```python
from build123d import *

# Parameters (mm, degrees)
F2_R     = 4.7625
F3_DEPTH = 5.08
F4_SIZE  = 0.381
F5_R     = 0.534423
F6_DEPTH = 25.4


with BuildPart() as f1:
    # F0 (on Front) → F1 (revolve)
    with BuildSketch(Plane.XZ):
        Polygon((0, 1.6002), (0, 0), (0, -3.2004), (12.659507, -3.2004), (12.659507, -1.6002), (10.346893, -1.6002), (10.346893, 0), (12.7, 0), (12.7, 1.6002), align=None)
    revolve(axis=Axis((0, 0, 0.8001), (0, 0, 1)))

    # F2 (on face) → F3 (cut)
    with BuildSketch(Plane.XY.offset(1.6002)):
        with Locations((0, -3.9624)):
            Circle(F2_R)
    extrude(amount=-F3_DEPTH, mode=Mode.SUBTRACT)

    # F4
    f4_edges = [f1.edges().sort_by_distance(p)[0] for p in [
        (-4.7625, -3.9624, 1.6002),
        (-12.7, 0, 1.6002),
        (-12.7, 0, 0),
        (-12.659507, 0, -1.6002),
        (-12.659507, 0, -3.2004),
        (-4.7625, -3.9624, -3.2004),
    ]]
    chamfer(f4_edges, length=F4_SIZE)

    # F5 (on Front) → F6 (cut)
    with BuildSketch(Plane.XZ):
        with Locations((0, -0.787439)):
            Circle(F5_R)
    extrude(amount=-F6_DEPTH, mode=Mode.SUBTRACT)


solid = f1.part
```
Work out the finished part from the listing and answer in its coordinate system (mm). A direction names the side the tool comes from. Round coordinates to 2 decimals unless told otherwise and drop trailing zeros. Write each question's results on one line, items separated by ' | '.
Q1. Determine the mould class of faces 1 (the cylindrical face through (9.87, 3.11, -0.79)), 2 (the cylindrical face through (-3.78, -6.86, -0.77)), 3 (the flat face through (0, 3, 1.6)) for opening direction X: released by +X, released by -X, zero draft, split by the parting line, or undercut.
Data:
face 1: split by the parting line | face 2: undercut | face 3: zero draft
Q2. Section A-A, the plane x = 0 is taken. Give the number of separate pieces and of enclosed holes in the cut face, then the cut area to 3 significant figures.
Data:
separate pieces: 3 | enclosed holes: 0 | area: 57.5 mm^2
Q3. Which of the six approach directions +Z, -Z, +X, -X, +Y, -Y give full straight-line access (tool end or side, diameter ignored) to faces 4 (the flat face through (0, 3, -3.2)), 5 (the cylindrical face through (-10.05, -7.7, -2.39)), 6 (the cylindrical face through (-0.12, 5.49, -1.31)), 7 (the flat face through (-6, -9, -1.6))?
Data:
face 4: -Z, +X, -X, +Y, -Y | face 5: -Z | face 6: +Y | face 7: none
Q4. Straight lines are drawn through the part: line 1 along Z through (x, y) = (11, -2.5); line 2 along Z through (x, y) = (0, 7.75); line 3 along Y through (x, z) = (0, -0.35). For each, find the intervals that lie inside material, in ascending order. Write a range as [from, to].
Data:
line 1: [-3.2, -1.6], [0, 1.6] | line 2: [-3.2, -1.32], [-0.25, 1.6] | line 3: [-10.35, -8.72]
Q5. Flat-ended cylindrical pins translate along their axes: P1, Ø2, axis at x = 9.5, z = 1, coming from the +Y side; P2, Ø1.7, axis at x = 0, z = -0.79, coming from the +Y side; P3, Ø1, axis at y = 8, z = -2, coming from the -X side. Find the tip coordinate at first contact, or state that the pin passes through.
Data:
P1: y = 9.44 | P2: y = 12.38 | P3: x = -10.2
